Build history of the part. All positions in model axes, mm. A direction names the side the tool comes from. Give positions to 0.01 mm unless a question says otherwise; leave off trailing zeros. Order: outer loops, then holes, each group sorted by start corner. A loop starts at its lowest first (then second) coordinate and runs counter-clockwise, first axis right, second up. Notation, with made-up numbers: (51, 4) -> (65, 4) arc R24 cw to (65, 35) -> close; hole circle Ø11 at (38, 53.25). An arc over 180 degrees is marked (long way). One line per item, written item: value. Start each with the question number.
(1) Saw through at A-A on x = 23.25. Give the cut face in (y, z), plus the area to 3 significant figures.
(2) Saw through at B-B on z = 8. Give the cut face in (x, y), plus the area to 3 significant figures.
(3) Which spindle directions (+Z, -Z, +X, -X, +Y, -Y) get a long thin tool onto all of the face, cutting with end or side? Do faces 4 (the flat face through (5, 31, -6)), 5 (the cylindrical face through (35.57, 2.46, -12.77)). Say none if no direction does.
(4) Saw through at C-C on x = 16.5. Give the cut face in (y, z).
(5) Saw through at D-D on y = 33. Give the cut face in (x, z).
(6) Pin check, flat tips, straight feed: pin 1 (2.5 mm diameter, centred on y = 26.56, z = -13.44, fed in from -X); pin 2 (18 mm diameter, centred on y = 51, z = -2, fed in from +X); pin 3 (4 mm diameter, centred on x = 23, z = -5.5, fed in from +Y). Stop position of each tip, or through.
(7) Two-plate mould, pull along Z, no slides. Class faces 1 (the flat face through (4, 13, -30)), 2 (the flat face through (26, 5, 0)), 3 (the cylindrical face through (23.99, 2.46, 13.11)): +Z half, -Z half, draft (parallel to the pull), parting line (faces both ways), or undercut.
(8) Probe line 1 (Z direction, x = 23, y = 1); line 2 (Z direction, x = 30, y = 3.45); line 3 (Z direction, x = 1.6, y = 40). List the from-to ranges inside material, lowest first.
```python
from build123d import *

# Parameters (mm, degrees)
SM_BASE_FLANGE_1_DEPTH  = 30
SKETCH_2_R              = 3.293373228
CUT_EXTRUDE_1_DEPTH     = 10
HOLE_WIZARD_1_OUTLINE_R = 1.6
HOLE_WIZARD_1_DEPTH     = 5
SKETCH_5_R              = 10
CUT_EXTRUDE_2_DEPTH     = 10
HOLE_WIZARD_2_OUTLINE_R = 1.6
HOLE_WIZARD_2_DEPTH     = 5
FILLET_1_R              = 30


# Read off the part's stored shape, not the designer's step: 孔1, 孔2
# Sheet-metal steps are written as plain solids
with BuildPart() as part:
    # Sketch 1 → 基体-法兰1 (new, symmetric)
    with BuildSketch(Plane.XY):
        with BuildLine():
            Line((60, 0), (5.7366, 0))
            ThreePointArc((5.7366, 0), (1.680211239, 1.680211239), (0, 5.7366))
            Line((0, 5.7366), (0, 70))
            Line((0, 70), (5, 70))
            Line((5, 70), (5, 5.7366))
            ThreePointArc((5, 5.7366), (5.215745145, 5.215745145), (5.7366, 5))
            Line((5.7366, 5), (60, 5))
            Line((60, 5), (60, 0))
        make_face()
    extrude(amount=SM_BASE_FLANGE_1_DEPTH, both=True)

    # Sketch 2 → 切除-拉伸1 (cut)
    with BuildSketch(Plane(origin=(0, 5, 0), x_dir=(1, 0, 0), z_dir=(0, 1, 0))):
        with Locations(Location((30, 0, 0), (0, 0, 180))):
            Circle(SKETCH_2_R)
    extrude(amount=-CUT_EXTRUDE_1_DEPTH, mode=Mode.SUBTRACT)

    # 孔1 outline → 孔1 (cut)
    with BuildSketch(Plane(origin=(0, 0, 0), x_dir=(1, 0, 0), z_dir=(0, 1, 0))):
        with Locations((23.25, -11.691342951)):
            Circle(HOLE_WIZARD_1_OUTLINE_R)
        with Locations((16.5, 0)):
            Circle(HOLE_WIZARD_1_OUTLINE_R)
        with Locations((23.25, 11.691342951)):
            Circle(HOLE_WIZARD_1_OUTLINE_R)
        with Locations((36.75, 11.691342951)):
            Circle(HOLE_WIZARD_1_OUTLINE_R)
        with Locations((43.5, 0)):
            Circle(HOLE_WIZARD_1_OUTLINE_R)
        with Locations((36.75, -11.691342951)):
            Circle(HOLE_WIZARD_1_OUTLINE_R)
    extrude(amount=HOLE_WIZARD_1_DEPTH, mode=Mode.SUBTRACT)

    # 草图5 → 切除-拉伸2 (cut)
    with BuildSketch(Plane.ZY):
        with Locations(Location((0, 40, 0), (0, 0, 270))):
            Circle(SKETCH_5_R)
    extrude(amount=-CUT_EXTRUDE_2_DEPTH, mode=Mode.SUBTRACT)

    # 孔2 outline → 孔2 (cut)
    with BuildSketch(Plane.YZ):
        with Locations((26.564971157, 13.435028843)):
            Circle(HOLE_WIZARD_2_OUTLINE_R)
        with Locations((26.564971157, -13.435028843)):
            Circle(HOLE_WIZARD_2_OUTLINE_R)
        with Locations((53.435028843, -13.435028843)):
            Circle(HOLE_WIZARD_2_OUTLINE_R)
        with Locations((53.435028843, 13.435028843)):
            Circle(HOLE_WIZARD_2_OUTLINE_R)
    extrude(amount=HOLE_WIZARD_2_DEPTH, mode=Mode.SUBTRACT)

    # 圆角1
    fillet_1_edges = [part.edges().sort_by_distance(p)[0] for p in [
        (60, 2.5, -30),
        (60, 2.5, 30),
        (2.5, 70, -30),
        (2.5, 70, 30),
    ]]
    fillet(fillet_1_edges, radius=FILLET_1_R - 0.0001)  # a hair under: the kernel refuses the full size


solid = part.part
```
Results below:
1. outline: (0, -30) -> (5, -30) -> (5, -13.29) -> (0, -13.29) -> close; (0, -10.09) -> (5, -10.09) -> (5, 10.09) -> (0, 10.09) -> close; (0, 13.29) -> (5, 13.29) -> (5, 30) -> (0, 30) -> close
1. area: 268 mm²
2. outline: (0, 5.74) arc R5.74 ccw to (5.74, 0) -> (58.91, 0) -> (58.91, 5) -> (5.74, 5) arc R0.74 cw to (5, 5.74) -> (5, 34) -> (0, 34) -> close; (0, 46) -> (5, 46) -> (5, 68.91) -> (0, 68.91) -> close
2. area: 547 mm²
3. face 4: +Z, -Z, +X, +Y
3. face 5: +Y, -Y
4. outline: (0, -30) -> (5, -30) -> (5, -1.6) -> (0, -1.6) -> close; (0, 1.6) -> (5, 1.6) -> (5, 30) -> (0, 30) -> close
5. outline: (0, -30) -> (5, -30) -> (5, -7.14) -> (0, -7.14) -> close; (0, 7.14) -> (5, 7.14) -> (5, 30) -> (0, 30) -> close
6. pin 1: passes through
6. pin 2: stops at x = 5
6. pin 3: stops at y = 5
7. face 1: -Z half
7. face 2: draft
7. face 3: undercut
8. line 1: z = -30 to -13.27, -10.11 to 10.11, 13.27 to 30
8. line 2: z = -30 to -3.29, 3.29 to 30
8. line 3: z = -30 to -10, 10 to 30
